Build history of the part. All positions in model axes, mm. Coordinates: 2 decimals unless noted, no trailing zeros. Order: outer loops, then holes, each group sorted by start corner. A loop starts at its lowest first (then second) coordinate and runs counter-clockwise, first axis right, second up. Notation, with made-up numbers: (56, 35.5) - (99, 35.5) arc R9 ccw to (99, 40.5) - close; hole circle Ø1 at (-37, -20.5). An arc over 180 degrees is marked (long way). One line per item, written item: value.
Autodesk Inventor part; units mm, degrees
ref_plane "YZ Plane" through (0, 0, 0) normal (1, 0, 0) x (0, 1, 0)
ref_plane "XZ Plane" through (0, 0, 0) normal (0, 1, 0) x (-1, 0, 0)
ref_plane "XY Plane" through (0, 0, 0) normal (0, 0, 1) x (1, 0, 0)
sketch "Sketch1" plane through (0, 0, 0) normal (0, 0, 1) x (1, 0, 0)
  circle A0 centre (0, 0) radius 11.25
  circle A1 centre (0, 0) radius 35.025
  circle A2 centre (0, 0) radius 37.030393
  arc A3 (-32.79294, -17.200962) -> (-31.29294, -19.799038) centre (0, 0) ccw
  line L0 (-32.79294, -17.200962) -> (-31.05471, -16.197395)
  line L1 (-32.79294, -17.200962) -> (-31.05471, -16.197395)
  line L2 (-29.55471, -18.795471) -> (-31.29294, -19.799038)
  line L3 (-31.29294, -19.799038) -> (-29.55471, -18.795471)
  line L4 (-16.197395, -31.05471) -> (-17.200962, -32.79294)
  line L5 (-17.200962, -32.79294) -> (-16.197395, -31.05471)
  arc A4 (-19.799038, -31.29294) -> (-17.200962, -32.79294) centre (0, 0) ccw
  line L6 (-19.799038, -31.29294) -> (-18.795471, -29.55471)
  line L7 (-19.799038, -31.29294) -> (-18.795471, -29.55471)
  arc A5 (17.200962, -32.79294) -> (19.799038, -31.29294) centre (0, 0) ccw
  line L8 (17.200962, -32.79294) -> (16.197395, -31.05471)
  line L9 (17.200962, -32.79294) -> (16.197395, -31.05471)
  line L10 (18.795471, -29.55471) -> (19.799038, -31.29294)
  line L11 (19.799038, -31.29294) -> (18.795471, -29.55471)
  arc A6 (31.29294, -19.799038) -> (32.79294, -17.200962) centre (0, 0) ccw
  line L12 (31.29294, -19.799038) -> (29.55471, -18.795471)
  line L13 (31.05471, -16.197395) -> (32.79294, -17.200962)
  line L14 (32.79294, -17.200962) -> (31.05471, -16.197395)
  line L15 (32.79294, 17.200962) -> (31.05471, 16.197395)
  line L16 (32.79294, 17.200962) -> (31.05471, 16.197395)
  arc A7 (32.79294, 17.200962) -> (31.29294, 19.799038) centre (0, 0) ccw
  line L17 (29.55471, 18.795471) -> (31.29294, 19.799038)
  line L18 (31.29294, 19.799038) -> (29.55471, 18.795471)
  line L19 (16.197395, 31.05471) -> (17.200962, 32.79294)
  line L20 (17.200962, 32.79294) -> (16.197395, 31.05471)
  line L21 (19.799038, 31.29294) -> (18.795471, 29.55471)
  line L22 (19.799038, 31.29294) -> (18.795471, 29.55471)
  line L23 (-17.200962, 32.79294) -> (-16.197395, 31.05471)
  line L24 (-17.200962, 32.79294) -> (-16.197395, 31.05471)
  line L25 (-18.795471, 29.55471) -> (-19.799038, 31.29294)
  line L26 (-19.799038, 31.29294) -> (-18.795471, 29.55471)
  arc A8 (-31.29294, 19.799038) -> (-32.79294, 17.200962) centre (0, 0) ccw
  line L27 (-31.29294, 19.799038) -> (-29.55471, 18.795471)
  line L28 (-31.29294, 19.799038) -> (-29.55471, 18.795471)
  line L29 (-31.05471, 16.197395) -> (-32.79294, 17.200962)
  line L30 (-32.79294, 17.200962) -> (-31.05471, 16.197395)
  arc A9 (-34.800207, -3.961848) -> (-34.800207, 3.961848) centre (-31.75, 0) ccw
  circle A10 centre (-31.75, 0) radius 5
  arc A11 (-3.961848, 34.800207) -> (3.961848, 34.800207) centre (0, 31.75) ccw
  circle A12 centre (0, 31.75) radius 5
  circle A13 centre (31.75, 0) radius 5
  circle A14 centre (31.75, 0) radius 5
  arc A15 (-3.961848, -34.800207) -> (3.961848, -34.800207) centre (0, -31.75) ccw
  circle A16 centre (0, -31.75) radius 5
  circle A17 centre (0, 31.75) radius 4.75
  circle A18 centre (-31.75, 0) radius 4.75
  circle A19 centre (0, -31.75) radius 4.75
  circle A20 centre (31.75, 0) radius 4.75
  circle A21 centre (0, 0) radius 34.775
  circle A22 centre (0, 0) radius 36.75
  point P0 (0, 0)
  point P1 (0, 49.75)
  point P2 (34.563789, -3.82689)
  point P3 (34.563789, 3.82689)
  point P4 (3.82689, 34.563789)
  point P5 (-3.82689, 34.563789)
  point P6 (-34.563789, 3.82689)
  point P7 (-34.563789, -3.82689)
  point P8 (-3.82689, -34.563789)
  point P9 (3.82689, -34.563789)
  dimension "d6" = 70.05
  dimension "d8" = 74.06079
  dimension "d0" = 10
  dimension "d1" = 0.25
  dimension "d4" = 360
  dimension "d7" = 0.25
  dimension "d9" = 73.5
sketch "Sketch1 outline for Extrusion1" plane through (0, 0, 0) normal (0, 0, 1) x (1, 0, 0)
  arc A0 (3.82689, -34.563789) -> (34.563789, -3.82689) centre (0, 0) ccw
  arc A1 (-3.82689, -34.563789) -> (3.82689, -34.563789) centre (0, -31.75) ccw
  arc A2 (-34.563789, -3.82689) -> (-3.82689, -34.563789) centre (0, 0) ccw
  arc A3 (-34.563789, 3.82689) -> (-34.563789, -3.82689) centre (-31.75, 0) ccw
  arc A4 (-3.82689, 34.563789) -> (-34.563789, 3.82689) centre (0, 0) ccw
  arc A5 (3.82689, 34.563789) -> (-3.82689, 34.563789) centre (0, 31.75) ccw
  arc A6 (34.563789, 3.82689) -> (3.82689, 34.563789) centre (0, 0) ccw
  arc A7 (34.563789, -3.82689) -> (34.563789, 3.82689) centre (31.75, 0) ccw
extrude "Extrusion1" add sketch "Sketch1 outline for Extrusion1" along normal blind 21.9
properties part number "dummy_blende_130x130x130mm_corpus"
1. Band-saw the part on B-B, the plane y = 13. Give the cut face in (x, z), and give its area (3 significant figures).
Values found:
outline: (-32.25, 0) - (32.25, 0) - (32.25, 21.9) - (-32.25, 21.9) - close
area: 1,410 mm2
2. Band-saw the part on C-C, the plane x = -23. Give the cut face in (y, z).
Values found:
outline: (-26.08, 0) - (26.08, 0) - (26.08, 21.9) - (-26.08, 21.9) - close
3. Flat gauge pins, fed straight in: P1, Ø8, axis at x = 7.5, z = 3.5, coming from the +Y side; P2, Ø3, axis at x = 16, z = 7, coming from the -Y side; P3, Ø3, axis at y = 28, z = 10.5, coming from the +X side. Where does each tip first touch, or does it go through?
Values found:
P1: stops at y = 34.96
P2: stops at y = -31.61
P3: stops at x = 22.52
4. Band-saw the part on A-A, the plane z = 8.5. Give the cut face in (x, y) (3 decimals).
Values found:
outline: (-34.564, -3.827) arc R34.775 ccw to (-3.827, -34.564) arc R4.75 ccw to (3.827, -34.564) arc R34.775 ccw to (34.564, -3.827) arc R4.75 ccw to (34.564, 3.827) arc R34.775 ccw to (3.827, 34.564) arc R4.75 ccw to (-3.827, 34.564) arc R34.775 ccw to (-34.564, 3.827) arc R4.75 ccw to start
5. Probe line 1 along Y through (x, z) = (7, 4.5); line 2 along X through (y, z) = (5.5, 11); line 3 along X through (y, z) = (-20, 11.75). List the from-to ranges inside material, lowest first.
Values found:
line 1: y = -34.06 to 34.06
line 2: x = -34.34 to 34.34
line 3: x = -28.45 to 28.45
